from build123d import *

# Parameters (mm, degrees)
SKETCH1_W             = 25
SKETCH1_H             = 5
BOSS_EXTRUDE1_DEPTH   = 6
BOSS_EXTRUDE1_2_DEPTH = 6
SKETCH2_W             = 42
SKETCH2_H             = 128
SKETCH2_W_2           = 34
SKETCH2_H_2           = 120
BOSS_EXTRUDE2_DEPTH   = 3
SKETCH2_3_W           = 34
SKETCH2_3_H           = 120
SKETCH2_3_R           = 16
BOSS_EXTRUDE3_DEPTH   = 2


with BuildPart() as part:
    # Sketch1 → Boss-Extrude1 (new body)
    with BuildSketch(Plane.XY):
        with Locations((0, -27.19848481)):
            Rectangle(SKETCH1_W, SKETCH1_H)
    extrude(amount=BOSS_EXTRUDE1_DEPTH)



with BuildPart() as body_2:
    # Sketch1 → Boss-Extrude1 2 (new body)
    with BuildSketch(Plane.XY):
        with Locations((0, 27.19848481)):
            Rectangle(SKETCH1_W, SKETCH1_H)
    extrude(amount=BOSS_EXTRUDE1_2_DEPTH)


with BuildPart() as body_3:
    # Sketch2 → Boss-Extrude2 (new body)
    with BuildSketch(Plane.XY.offset(6)):
        Rectangle(SKETCH2_W, SKETCH2_H)
        Rectangle(SKETCH2_W_2, SKETCH2_H_2, mode=Mode.SUBTRACT)
    extrude(amount=-BOSS_EXTRUDE2_DEPTH)


with BuildPart() as part_1:
    add(part.part)

    add(body_2.part)  # Boss-Extrude3 merges body 2

    add(body_3.part)  # Boss-Extrude3 merges body 3
    # Sketch2_3 → Boss-Extrude3 (add)
    with BuildSketch(Plane.XY.offset(6)):
        Rectangle(SKETCH2_3_W, SKETCH2_3_H)
        with Locations((0, -42)):
            Circle(SKETCH2_3_R, mode=Mode.SUBTRACT)
        with Locations((0, 42)):
            Circle(SKETCH2_3_R, mode=Mode.SUBTRACT)
        Circle(SKETCH2_3_R, mode=Mode.SUBTRACT)
    extrude(amount=-BOSS_EXTRUDE3_DEPTH)


solid = part_1.part
Geometry check sheet. Reference: the model listing, model coordinates, mm. A direction names the side the tool comes from. Coordinates: 2 decimals unless noted, no trailing zeros. Write each loop counter-clockwise with the first axis right and the second up, starting at its lowest first coordinate (ties: lowest second). Pieces come first, ordered by that corner, then holes. Notation, with made-up numbers: (45.5, 65) -> (99.5, 65) arc R17 cw to (99.5, 76) -> close; hole circle Ø6 at (-6.5, 51). An arc over 180 degrees is marked (long way). One line per question, with ' | ' between items.
1. Cross-section at C-C on y = 47. Record the cut outline in (x, z).
Answers:
outline: (-21, 3) -> (-17, 3) -> (-17, 4) -> (-15.2, 4) -> (-15.2, 6) -> (-21, 6) -> close; (15.2, 4) -> (17, 4) -> (17, 3) -> (21, 3) -> (21, 6) -> (15.2, 6) -> close
2. Draft check along X on faces 3 (the flat face through (-12.5, -27, 2)), 4 (the flat face through (-21, -1, 5)), 5 (the flat face through (0, -27, 0)). Enter one of: +X half, -X half, draft (parallel to the pull), parting line (faces both ways), or undercut.
Answers:
face 3: undercut | face 4: -X half | face 5: draft
3. Set-up check for faces 1 (the flat face through (12.5, -27, 2)), 2 (the flat face through (21, -1, 5)): record each of +Z, -Z, +X, -X, +Y, -Y from which the full face is reachable in a straight line by a thin tool's end or side.
Answers:
face 1: -Z | face 2: +Z, -Z, +X, +Y, -Y
4. Depth check by flat-ended pin: pin 1 Ø3 at (y, z) = (-28, 1) entering from -X; pin 2 Ø1.2 at (x, z) = (5, 2.5) entering from -Y; pin 3 Ø12.5 at (x, y) = (-6, -14) entering from -Z. Enter the tip coordinate at first touch or a pass-through.
Answers:
pin 1: stops at x = -12.5 | pin 2: stops at y = -64 | pin 3: stops at z = 4
5. Cross-section at A-A on y = -42. Record the cut outline in (x, z), and give its area (3 significant figures).
Answers:
outline: (-21, 3) -> (-17, 3) -> (-17, 4) -> (-16, 4) -> (-16, 6) -> (-21, 6) -> close; (16, 4) -> (17, 4) -> (17, 3) -> (21, 3) -> (21, 6) -> (16, 6) -> close | area: 28.0 mm²
6. Thickness scan on probe 1 along Y at (x, z) = (0, 4.8); probe 2 along Y at (x, z) = (1.5, 1.45); probe 3 along Y at (x, z) = (-13, 5.15). Record the ranges inside material, lowest first. Write a range as from..to.
Answers:
probe 1: y = -64..-58, -29.7..-16, 16..29.7, 58..64 | probe 2: y = -29.7..-24.7, 24.7..29.7 | probe 3: y = -64..-51.33, -32.67..-9.33, 9.33..32.67, 51.33..64
7. Cross-section at B-B on y = -20. Record the cut outline in (x, z), and give its area (3 significant figures).
Answers:
outline: (-21, 3) -> (-17, 3) -> (-17, 4) -> (17, 4) -> (17, 3) -> (21, 3) -> (21, 6) -> (-21, 6) -> close | area: 92.0 mm²
